```python
from build123d import *

# Parameters (mm, degrees)
SKETCH1_W           = 127
SKETCH1_H           = 52.832
BOSS_EXTRUDE1_DEPTH = 4.7625
FILLET1_R           = 2.54
SKETCH2_R           = 2.69
CUT_EXTRUDE1_DEPTH  = 69.940093286


with BuildPart() as part:
    # Sketch1 → Boss-Extrude1 (new body)
    with BuildSketch(Plane(origin=(0, 0, 0), x_dir=(1, 0, 0), z_dir=(0, 1, 0))):
        Rectangle(SKETCH1_W, SKETCH1_H)
    extrude(amount=BOSS_EXTRUDE1_DEPTH)

    # Fillet1
    fillet1_edges = [part.edges().sort_by_distance(p)[0] for p in [
        (63.5, 2.38125, 26.416),
        (-63.5, 2.38125, 26.416),
        (-63.5, 2.38125, -26.416),
        (63.5, 2.38125, -26.416),
    ]]
    fillet(fillet1_edges, radius=FILLET1_R)

    # Sketch2 → Cut-Extrude1 (cut, through all)
    with BuildSketch(Plane.XZ):
        with Locations(Location((57.15, -15.24, 0), (0, 0, 270))):
            Circle(SKETCH2_R)
        with Locations(Location((57.15, 0, 0), (0, 0, 270))):
            Circle(SKETCH2_R)
        with Locations(Location((57.15, 15.24, 0), (0, 0, 270))):
            Circle(SKETCH2_R)
    cut_extrude1 = extrude(amount=-CUT_EXTRUDE1_DEPTH, mode=Mode.SUBTRACT)

    # Mirror1: Cut-Extrude1 across plane
    add(cut_extrude1.mirror(Plane(origin=(0, 0, 0), x_dir=(0, 0, 1), z_dir=(1, 0, 0))), mode=Mode.SUBTRACT)


solid = part.part
```
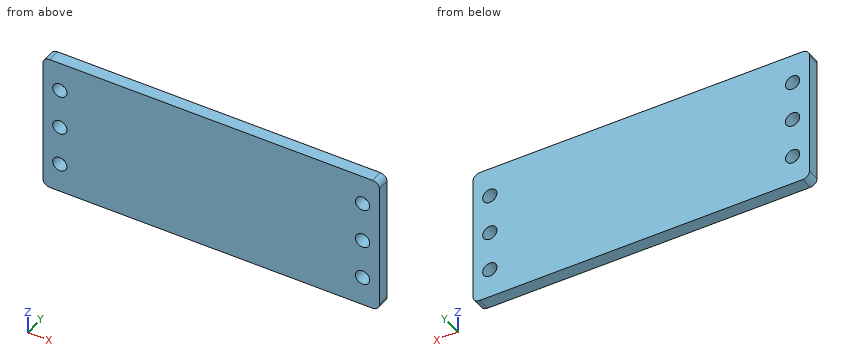
For this review, take the finished solid that the model builds, in its own axes (mm). Round coordinates to 2 decimals unless told otherwise and drop trailing zeros. Write each loop counter-clockwise with the first axis right and the second up, starting at its lowest first coordinate (ties: lowest second). Pieces come first, ordered by that corner, then holes. Notation, with made-up numbers: (50.25, 76.5) -> (75.25, 76.5) arc R8 cw to (75.25, 88.5) -> close; hole circle Ø5 at (9, 75). An arc over 180 degrees is marked (long way). One line per question, with ' | ' between items. Start each with the question number.
1) Add section C-C (x = 57.15). Write out the cut boundary in (y, z), and give its area (3 significant figures).
2) Wall thickness on line 1 along X through (y, z) = (2.1, 0); line 2 along Z through (x, y) = (-57.15, 3.4); line 3 along X through (y, z) = (0.95, -16.5): over which ranges is each line inside the solid? List them lowest first.
3) Add section A-A (z = -15.24). Write out the cut boundary in (x, y), and give its area (3 significant figures).
4) Add section B-B (y = 3.55). Write out the cut boundary in (x, z), and give its area (3 significant figures).
5) For pin 1 Ø8.5 at (x, z) = (-57.15, 0) entering from -Y, flat-tipped, find the tip position at first contact; note if it passes through.
Reported:
1) outline: (0, -26.42) -> (4.76, -26.42) -> (4.76, -17.93) -> (0, -17.93) -> close; (0, -12.55) -> (4.76, -12.55) -> (4.76, -2.69) -> (0, -2.69) -> close; (0, 2.69) -> (4.76, 2.69) -> (4.76, 12.55) -> (0, 12.55) -> close; (0, 17.93) -> (4.76, 17.93) -> (4.76, 26.42) -> (0, 26.42) -> close | area: 175 mm²
2) line 1: x = -63.5 to -59.84, -54.46 to 54.46, 59.84 to 63.5 | line 2: z = -26.42 to -17.93, -12.55 to -2.69, 2.69 to 12.55, 17.93 to 26.42 | line 3: x = -63.5 to -59.53, -54.77 to 54.77, 59.53 to 63.5
3) outline: (-63.5, 0) -> (-59.84, 0) -> (-59.84, 4.76) -> (-63.5, 4.76) -> close; (-54.46, 0) -> (54.46, 0) -> (54.46, 4.76) -> (-54.46, 4.76) -> close; (59.84, 0) -> (63.5, 0) -> (63.5, 4.76) -> (59.84, 4.76) -> close | area: 554 mm²
4) outline: (-63.5, -23.88) arc R2.54 ccw to (-60.96, -26.42) -> (60.96, -26.42) arc R2.54 ccw to (63.5, -23.88) -> (63.5, 23.88) arc R2.54 ccw to (60.96, 26.42) -> (-60.96, 26.42) arc R2.54 ccw to (-63.5, 23.88) -> close; hole circle Ø5.38 at (-57.15, -15.24); hole circle Ø5.38 at (-57.15, 0); hole circle Ø5.38 at (-57.15, 15.24); hole circle Ø5.38 at (57.15, -15.24); hole circle Ø5.38 at (57.15, 0); hole circle Ø5.38 at (57.15, 15.24) | area: 6,570 mm²
5) pin 1: stops at y = 0
